Check sheet for the modelled part. Datum: model origin and axes. Units: mm. Face numbers are marked on the shaded views. A direction names the side the tool comes from. Round coordinates to 2 decimals unless told otherwise and drop trailing zeros. Order: outer loops, then holes, each group sorted by start corner. A loop starts at its lowest first (then second) coordinate and runs counter-clockwise, first axis right, second up. Notation, with made-up numbers: (24, 5.25) -> (41, 5.25) arc R36 ccw to (41, 41.25) -> close; hole circle Ø11 at (49.25, 45.5). An arc over 180 degrees is marked (long way). Answer in a Markdown table with one row per item. Add a question column.
1. Sectioned sample at B-B, the plane z = 7. Record the boundary of the cut face in (x, y).
2. Depth check by flat-ended pin: P1, Ø1, axis at y = 20, z = 15, coming from the -X side; P2, Ø6.5, axis at x = 1.5, y = 18, coming from the +Z side. Enter the tip coordinate at first touch or a pass-through.
3. Access from +Z, -Z, +X, -X, +Y, -Y to the whole of each face (thin tool, end or side, straight path). Record for the marked faces 1 and 2.
4. Material ranges on L1, parallel to Y at x = -6.5, z = 42.5; L2, parallel to X at y = 15, z = 23.5; L3, parallel to Y at x = 1.5, z = 23.5, recorded low to high. Write a range as from..to.
5. Sectioned sample at C-C, the plane y = 21. Record the boundary of the cut face in (x, z).
6. Sectioned sample at D-D, the plane x = 8.5. Record the boundary of the cut face in (y, z), then the cut area to 3 significant figures.
7. Sectioned sample at A-A, the plane x = 3.75. Record the boundary of the cut face in (y, z).
```python
from build123d import *

# Parameters (mm, degrees)
F1_DEPTH = 25.4
F0_W     = 25.4
F0_H     = 25.4
F2_DEPTH = 50.8


with BuildPart() as f1:
    # F0 (on Top) → F1 (new body)
    with BuildSketch(Plane.XY):
        Polygon((-12.7, 12.7), (12.7, 12.7), (0, 25.4), align=None)
    extrude(amount=F1_DEPTH)

    # F0 (on Top) → F2 (join)
    with BuildSketch(Plane.XY):
        Rectangle(F0_W, F0_H)
    extrude(amount=F2_DEPTH)


solid = f1.part
```
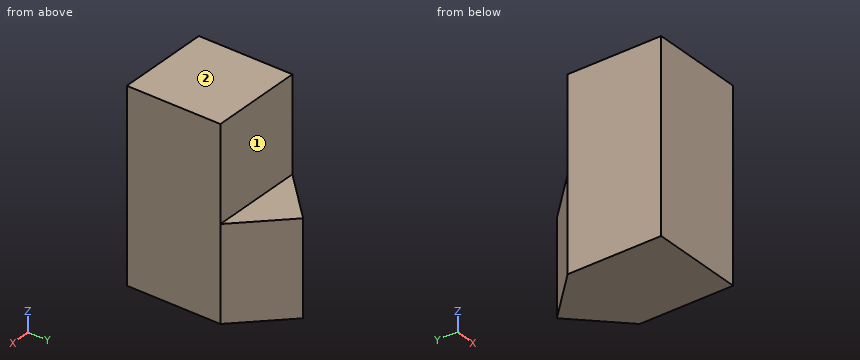
Answer key:
| question | item | result |
|---|---|---|
| 1 | outline | (-12.7, -12.7) -> (12.7, -12.7) -> (12.7, 12.7) -> (0, 25.4) -> (-12.7, 12.7) -> close |
| 2 | P1 | stops at x = -5.9 |
| 2 | P2 | stops at z = 25.4 |
| 3 | face 1 | +Z, +X, -X, +Y |
| 3 | face 2 | +Z, +X, -X, +Y, -Y |
| 4 | L1 | y = -12.7..12.7 |
| 4 | L2 | x = -10.4..10.4 |
| 4 | L3 | y = -12.7..23.9 |
| 5 | outline | (-4.4, 0) -> (4.4, 0) -> (4.4, 25.4) -> (-4.4, 25.4) -> close |
| 6 | outline | (-12.7, 0) -> (16.9, 0) -> (16.9, 25.4) -> (12.7, 25.4) -> (12.7, 50.8) -> (-12.7, 50.8) -> close |
| 6 | area | 1,400 mm² |
| 7 | outline | (-12.7, 0) -> (21.65, 0) -> (21.65, 25.4) -> (12.7, 25.4) -> (12.7, 50.8) -> (-12.7, 50.8) -> close |
